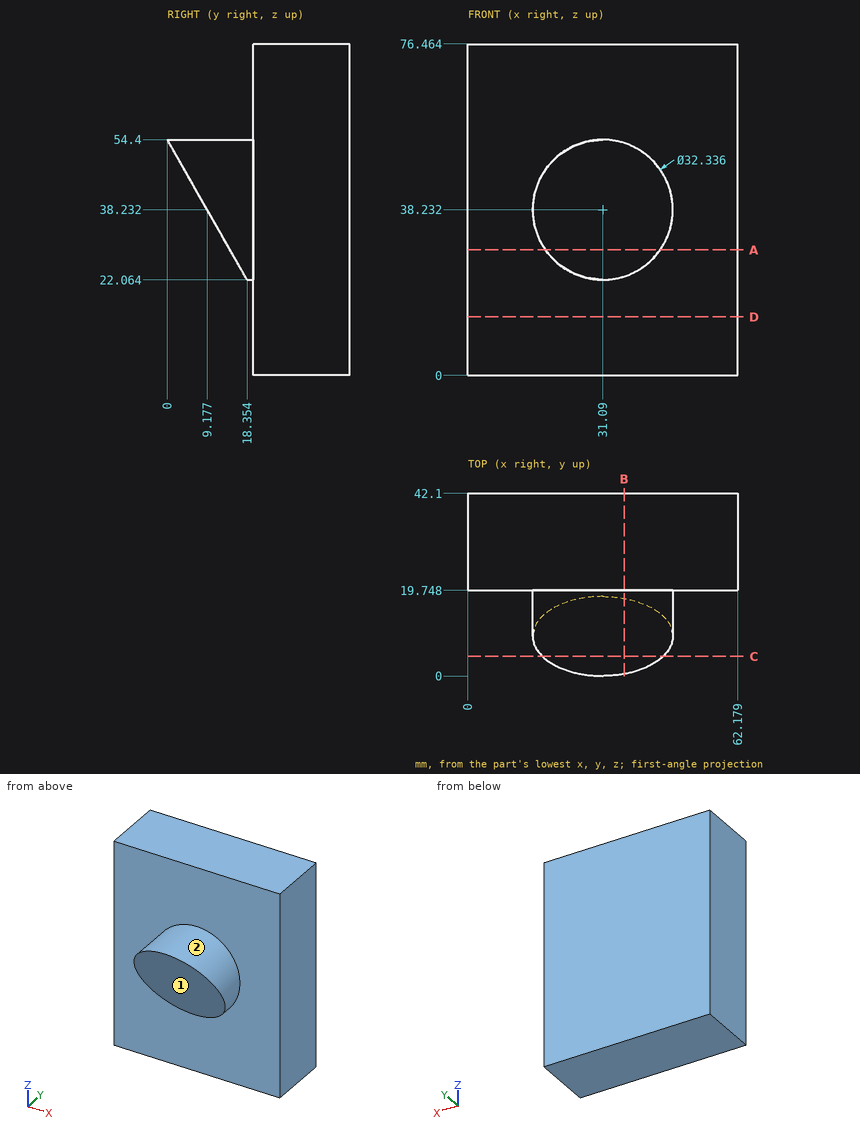
Can you work these out from the drawing? Everything is in mm from the part's minimum corner. A direction names the side the tool comes from. Round coordinates to 2 decimals unless told otherwise and drop trailing zeros. Loops run counter-clockwise (first coordinate to the right, second up) from the corner with the lowest first, then second, coordinate; pieces in that order, holes last. Notation, with made-up numbers: M 53,1 L 67,1 A26 ccw 67,27 Z; hole C 68.25,3.5 d6. An arc over 180 degrees is marked long. Write item = value, one per line.
1. I want a section at B-B, the plane x = 36. Write out the boundary of the cut face in (y, z), and give its area (3 significant figures).
Results below:
outline = M 0.43,53.64 L 17.92,22.83 L 19.75,22.83 L 19.75,0 L 42.1,0 L 42.1,76.46 L 19.75,76.46 L 19.75,53.64 Z
area = 2,030 mm²
2. I need wall thicknesses on probe 1 along Y at (x, z) = (7.5, 59); probe 2 along X at (y, z) = (16, 37.5); probe 3 along Y at (x, z) = (17, 39). Which ranges of each line are inside material? Lowest first, please.
Results below:
probe_1 = 19.75 to 42.1
probe_2 = 14.94 to 47.24
probe_3 = 8.74 to 42.1
3. Will these pins go through, and if not, where does the flat tip stop? P1, Ø2, axis at x = 23, y = 17, coming from the -Z side; P2, Ø18.5, axis at x = 27.5, z = 24.5, coming from the -Y side; P3, Ø6, axis at x = 53, z = 45, coming from the -Y side.
Results below:
P1 = 23.74
P2 = 11.72
P3 = 19.75
4. Which directions (+Z, -Z, +X, -X, +Y, -Y) give clear straight access to the entire face, cutting with the end or side of a thin tool? Please do the marked faces 1 and 2.
Results below:
face_1 = -Z, +X, -X, -Y
face_2 = -Y
5. I want a section at D-D, the plane z = 13.5. Write out the boundary of the cut face in (x, y).
Results below:
outline = M 0,19.75 L 62.18,19.75 L 62.18,42.1 L 0,42.1 Z
6. I want a section at A-A, the plane z = 29. Write out the boundary of the cut face in (x, y), and give its area (3 significant figures).
Results below:
outline = M 0,19.75 L 17.82,19.75 L 17.82,14.42 L 44.36,14.42 L 44.36,19.75 L 62.18,19.75 L 62.18,42.1 L 0,42.1 Z
area = 1,530 mm²
7. I want a section at C-C, the plane y = 4.5. Write out the boundary of the cut face in (x, z), and give its area (3 significant figures).
Results below:
outline = M 17.18,46.47 L 45,46.47 A16.17 ccw Z
area = 156 mm²
